The drawing under review shows one solid part. Ordinate dimensions are in mm from its lowest x, y, z. A direction names the side the tool comes from. Coordinates: 2 decimals unless noted, no trailing zeros. Write each loop counter-clockwise with the first axis right and the second up, starting at its lowest first coordinate (ties: lowest second). Pieces come first, ordered by that corner, then holes.
Q1. The part is to be moulded in two halves that separate along X. For the marked faces 3, 4 and 5, say which applies: +X half, -X half, draft (parallel to the pull), parting line (faces both ways), or undercut.
Q2. Add section D-D, the plane z = 28.5. Give the boundary of the cut face in (x, y).
Q3. Add section C-C, the plane x = 13. Give the boundary of the cut face in (y, z).
Q4. To check wall thickness, follow probe 1 along Y at (x, z) = (17.5, 39); probe 2 along Y at (x, z) = (20, 21); probe 3 along Y at (x, z) = (18, 40.5). State the ranges of each line that lie inside material, in increasing order.
Q5. Add section A-A, the plane x = 20. Give the boundary of the cut face in (y, z).
Q6. Machinability: for the marked faces 1 and 2, which of the approach directions +Z, -Z, +X, -X, +Y, -Y give a long, thin tool a straight path to every point of the face, cutting with its end or side? Answer none if there is none.
Q7. Add section B-B, the plane y = 24. Give the boundary of the cut face in (x, z), plus the area to 3 significant figures.
Q8. Clearance check with flat-ended pins moving along their axes: pin 1 Ø5 at (x, y) = (33.44, 37.44) entering from -Z; pin 2 Ø6.5 at (x, y) = (20, 5) entering from -Z; pin 3 Ø2 at (x, z) = (24, 34) entering from +Y; pin 4 Ø5 at (x, z) = (18.5, 16) entering from +Y. State where each tip first meets the part, or that it passes through.
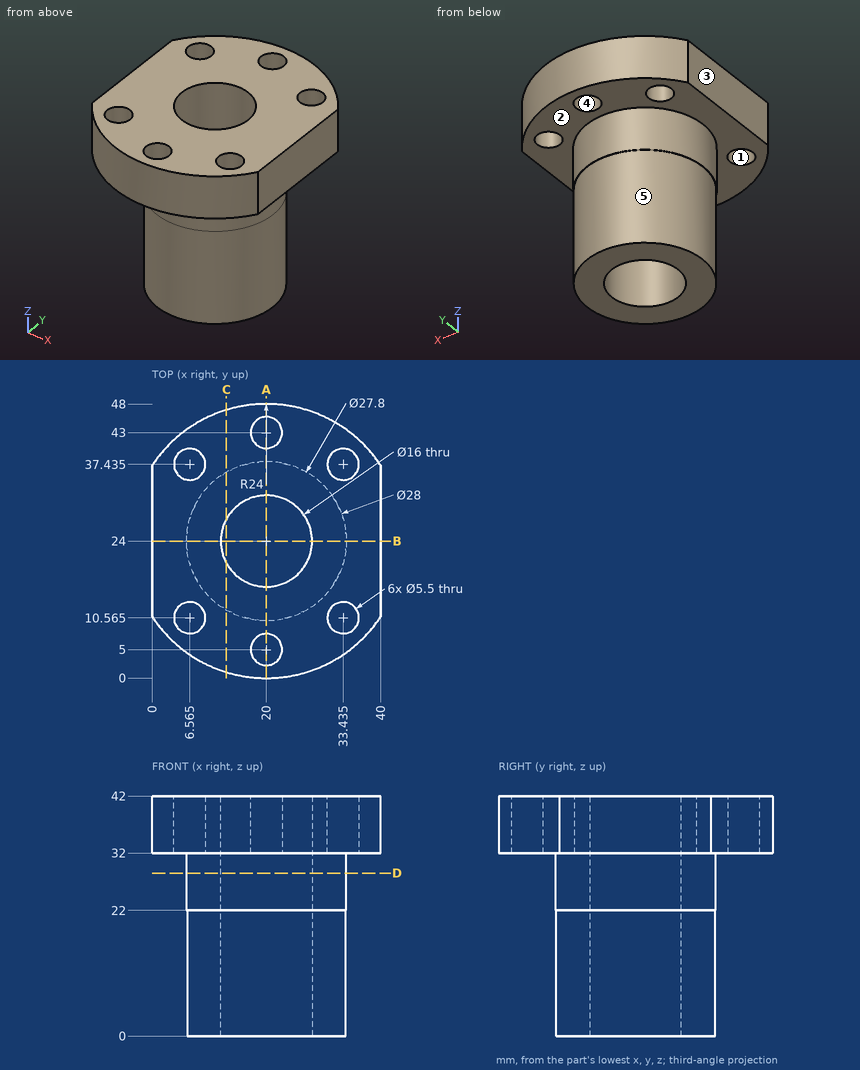
Here are the results:
1. face 3: -X half
1. face 4: undercut
1. face 5: parting line
2. outline: circle Ø28 at (20, 24); hole circle Ø16 at (20, 24)
3. outline: (1.04, 32) - (11.88, 32) - (11.88, 22) - (11.99, 22) - (11.99, 0) - (20.13, 0) - (20.13, 42) - (1.04, 42) - close; (27.87, 0) - (36.01, 0) - (36.01, 22) - (36.12, 22) - (36.12, 32) - (46.96, 32) - (46.96, 42) - (27.87, 42) - close
4. probe 1: y = 0.13 to 3.85, 6.15 to 16.4, 31.6 to 41.85, 44.15 to 47.87
4. probe 2: y = 10.1 to 16, 32 to 37.9
4. probe 3: y = 0.08 to 3.11, 6.89 to 16.25, 31.75 to 41.11, 44.89 to 47.92
5. outline: (0, 32) - (2.25, 32) - (2.25, 42) - (0, 42) - close; (7.75, 32) - (10, 32) - (10, 22) - (10.1, 22) - (10.1, 0) - (16, 0) - (16, 42) - (7.75, 42) - close; (32, 0) - (37.9, 0) - (37.9, 22) - (38, 22) - (38, 32) - (40.25, 32) - (40.25, 42) - (32, 42) - close; (45.75, 32) - (48, 32) - (48, 42) - (45.75, 42) - close
6. face 1: +Z, -Z
6. face 2: -Z
7. outline: (0, 32) - (6, 32) - (6, 22) - (6.1, 22) - (6.1, 0) - (12, 0) - (12, 42) - (0, 42) - close; (28, 0) - (33.9, 0) - (33.9, 22) - (34, 22) - (34, 32) - (40, 32) - (40, 42) - (28, 42) - close
7. area: 620 mm2
8. pin 1: passes through
8. pin 2: stops at z = 32
8. pin 3: stops at y = 47.81
8. pin 4: stops at y = 37.9
